For this review, take the finished solid that the model builds, in its own axes (mm). A direction names the side the tool comes from. Coordinates: 2 decimals unless noted, no trailing zeros. Loops run counter-clockwise (first coordinate to the right, second up) from the corner with the lowest first, then second, coordinate; pieces in that order, holes last. Notation, with made-up numbers: (65, 53.25) -> (116, 53.25) arc R14 cw to (116, 62.25) -> close; hole circle Ø3 at (31, -14). An arc over 180 degrees is marked (long way). Use a Markdown table: item, result.
from build123d import *

# Parameters (mm, degrees)
BOSS_EXTRUDE1_DEPTH = 12


with BuildPart() as part:
    # Sketch1 → Boss-Extrude1 (new body)
    with BuildSketch(Plane.XY):
        with BuildLine():
            Line((-147.556413952, 174.626444756), (-101.192621764, 174.626444756))
            ThreePointArc((-101.192621764, 174.626444756), (-97.418155085, 174.138042833), (-97.917719368, 177.911048356))
            Line((-97.917719368, 177.911048356), (-97.917719368, 186.626444756))
            Line((-97.917719368, 186.626444756), (-47.917719368, 186.626444756))
            Line((-47.917719368, 186.626444756), (-47.917719368, 177.911048356))
            ThreePointArc((-47.917719368, 177.911048356), (-48.417283652, 174.138042833), (-44.642816972, 174.626444756))
            Line((-44.642816972, 174.626444756), (-1.192621764, 174.626444756))
            ThreePointArc((-1.192621764, 174.626444756), (2.581844915, 174.138042833), (2.082280632, 177.911048356))
            Line((2.082280632, 177.911048356), (2.082280632, 186.626444756))
            Line((2.082280632, 186.626444756), (52.082280632, 186.626444756))
            Line((52.082280632, 186.626444756), (52.082280632, 177.911048356))
            ThreePointArc((52.082280632, 177.911048356), (51.582716348, 174.138042833), (55.357183028, 174.626444756))
            Line((55.357183028, 174.626444756), (98.807378236, 174.626444756))
            ThreePointArc((98.807378236, 174.626444756), (102.581844915, 174.138042833), (102.082280632, 177.911048356))
            Line((102.082280632, 177.911048356), (102.082280632, 186.626444756))
            Line((102.082280632, 186.626444756), (152.082280632, 186.626444756))
            Line((152.082280632, 186.626444756), (152.082280632, 177.911048356))
            ThreePointArc((152.082280632, 177.911048356), (151.582716348, 174.138042833), (155.357183028, 174.626444756))
            Line((155.357183028, 174.626444756), (201.720975216, 174.626444756))
            Line((201.720975216, 174.626444756), (201.720975216, -174.373555244))
            Line((201.720975216, -174.373555244), (155.357183028, -174.373555244))
            ThreePointArc((155.357183028, -174.373555244), (151.582716348, -173.885153322), (152.082280632, -177.658158845))
            Line((152.082280632, -177.658158845), (152.082280632, -186.373555244))
            Line((152.082280632, -186.373555244), (102.082280632, -186.373555244))
            Line((102.082280632, -186.373555244), (102.082280632, -177.658158845))
            ThreePointArc((102.082280632, -177.658158845), (102.581844915, -173.885153322), (98.807378236, -174.373555244))
            Line((98.807378236, -174.373555244), (55.357183028, -174.373555244))
            ThreePointArc((55.357183028, -174.373555244), (51.582716348, -173.885153322), (52.082280632, -177.658158845))
            Line((52.082280632, -177.658158845), (52.082280632, -186.373555244))
            Line((52.082280632, -186.373555244), (2.082280632, -186.373555244))
            Line((2.082280632, -186.373555244), (2.082280632, -177.658158845))
            ThreePointArc((2.082280632, -177.658158845), (2.581844915, -173.885153322), (-1.192621764, -174.373555244))
            Line((-1.192621764, -174.373555244), (-44.642816972, -174.373555244))
            ThreePointArc((-44.642816972, -174.373555244), (-48.417283652, -173.885153322), (-47.917719368, -177.658158845))
            Line((-47.917719368, -177.658158845), (-47.917719368, -186.373555244))
            Line((-47.917719368, -186.373555244), (-97.917719368, -186.373555244))
            Line((-97.917719368, -186.373555244), (-97.917719368, -177.658158845))
            ThreePointArc((-97.917719368, -177.658158845), (-97.418155085, -173.885153322), (-101.192621764, -174.373555244))
            Line((-101.192621764, -174.373555244), (-147.556413952, -174.373555244))
            Line((-147.556413952, -174.373555244), (-147.556413952, 174.626444756))
        make_face()
    extrude(amount=BOSS_EXTRUDE1_DEPTH)


solid = part.part
(1) Mouldability with a two-part tool opening along X and no side actions: class faces 1 (the face through (-147.556, -2, 6)), 2 (the face through (27, -186.374, 6)), 3 (the face through (-47.918, -182, 6)) as pulls with the +X half, pulls with the -X half, needs draft (parallel to the pull), parting line crosses it, or undercut.
Found:
| item | result |
|---|---|
| face 1 | pulls with the -X half |
| face 2 | needs draft |
| face 3 | undercut |
(2) For faces 4 (the face through (-97.918, 182, 6)), 5 (the face through (52.082, -182, 6)), 6 (the face through (179, -174.374, 6)), 7 (the face through (52.082, 182, 6)), list the 3-axis set-ups (+Z, -Z, +X, -X, +Y, -Y) from which the entire face can be reached by the end or side of a thin tool; tool diameter is ignored.
Found:
| item | result |
|---|---|
| face 4 | +Z, -Z, -X, +Y |
| face 5 | +Z, -Z, -Y |
| face 6 | +Z, -Z, +X, -Y |
| face 7 | +Z, -Z, +Y |
(3) For pin 1 Ø3 at (x, y) = (-99.12, -175.58) entering from +Z; pin 2 Ø3.5 at (x, z) = (168, 8.5) entering from -Y; pin 3 Ø3 at (x, y) = (13, 143) entering from -Z; pin 4 Ø4.5 at (y, z) = (-181, 4) entering from -X, all flat-tipped, find the tip position at first contact; note any pin that passes through.
Found:
| item | result |
|---|---|
| pin 1 | passes through |
| pin 2 | stops at y = -174.37 |
| pin 3 | stops at z = 0 |
| pin 4 | stops at x = -97.92 |
(4) Take a section at A-A on x = -16.5. Write out the cut boundary in (y, z), plus the area to 3 significant figures.
Found:
| item | result |
|---|---|
| outline | (-174.37, 0) -> (174.63, 0) -> (174.63, 12) -> (-174.37, 12) -> close |
| area | 4,190 mm^2 |
(5) For line 1 along Y through (x, z) = (-17, 5.75), list the stretches that pass through material, from the lowest coordinate up.
Found:
| item | result |
|---|---|
| line 1 | y = -174.37 to 174.63 |
